Part print with two shaded views. Sizes in mm from the minimum x, y, z corner. Round coordinates to 2 decimals unless told otherwise and drop trailing zeros. Loops run counter-clockwise (first coordinate to the right, second up) from the corner with the lowest first, then second, coordinate; pieces in that order, holes last. Notation, with made-up numbers: (73, 13.25) -> (83, 13.25) arc R27 cw to (83, 37.25) -> close; hole circle Ø11 at (8.25, -24.5). An arc over 180 degrees is marked (long way). Use a Markdown table: item, result. Add a question column.
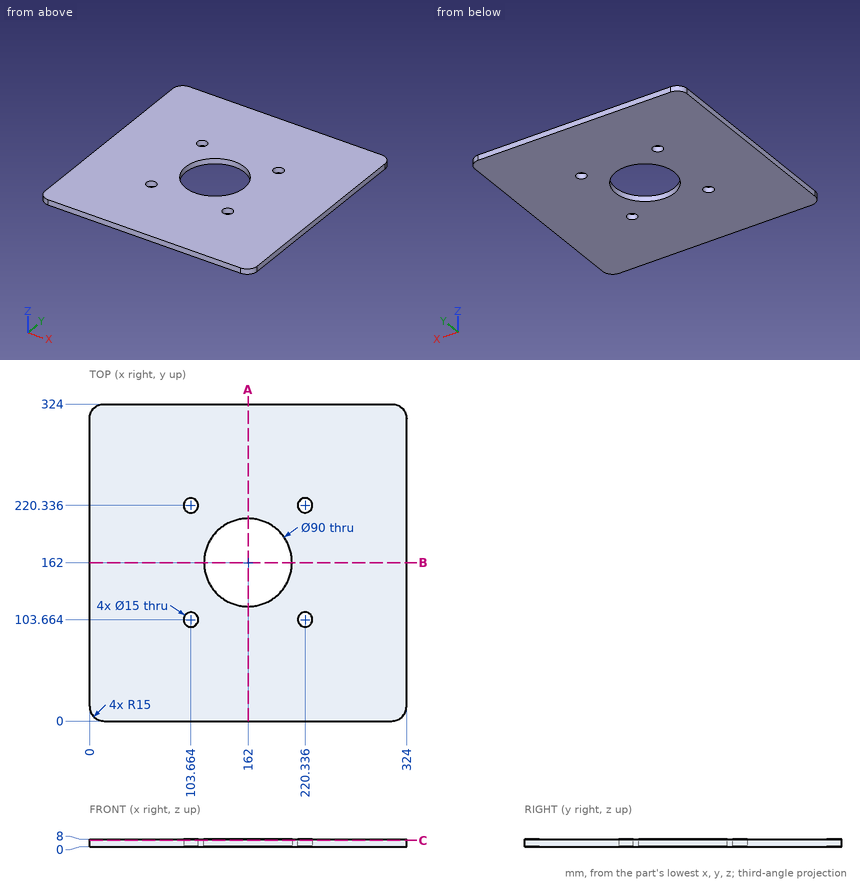
1) Cut at A-A on x = 162. Write the cut outline in (y, z), and give its area (3 significant figures).
2) Wall check: probe 1 along Y at (x, z) = (98, 2.75); probe 2 along Y at (x, z) = (162, 6); probe 3 along Y at (x, z) = (222, 4.25). Give the ranges that are in metal, low to high. Write a range as from..to.
3) Cut at C-C on z = 6.5. Write the cut outline in (x, y).
Established:
| question | item | result |
|---|---|---|
| 1 | outline | (0, 0) -> (117, 0) -> (117, 8) -> (0, 8) -> close; (207, 0) -> (324, 0) -> (324, 8) -> (207, 8) -> close |
| 1 | area | 1,870 mm^2 |
| 2 | probe 1 | y = 0..98.75, 108.58..215.42, 225.25..324 |
| 2 | probe 2 | y = 0..117, 207..324 |
| 2 | probe 3 | y = 0..96.35, 110.98..213.02, 227.65..324 |
| 3 | outline | (0, 15) arc R15 ccw to (15, 0) -> (309, 0) arc R15 ccw to (324, 15) -> (324, 309) arc R15 ccw to (309, 324) -> (15, 324) arc R15 ccw to (0, 309) -> close; hole circle Ø15 at (103.66, 103.66); hole circle Ø15 at (103.66, 220.34); hole circle Ø90 at (162, 162); hole circle Ø15 at (220.34, 103.66); hole circle Ø15 at (220.34, 220.34) |
